Autodesk Fusion 360 part; units mm, degrees
sketch "Skizze1" plane through (0, 0, 0) normal (0, 1, 0) x (1, 0, 0)
  line L0 (0, 75) -> (0, -65)
  line L1 (0, -50) -> (0, 75)
  line L2 (-85, 0) -> (95, 0)
  line L3 (0, 0) -> (-37.5, 0)
  line L4 (-37.5, 0) -> (-37.5, -25)
  line L5 (-37.5, -25) -> (0, -25)
  line L6 (0, -25) -> (0, 0)
  line L7 (37.5, 0) -> (37.5, -25)
  line L8 (37.5, -25) -> (0, -25)
  line L9 (-37.5, 0) -> (-37.5, 25)
  line L10 (-37.5, 25) -> (0, 25)
  line L11 (37.5, 25) -> (0, 25)
  line L12 (37.5, 0) -> (37.5, 25)
  line L13 (-25.2075, -10.9903) -> (-29.8263, -11.0098)
  line L14 (-29.8263, -11.0098) -> (-32.1188, -15.0195)
  line L15 (-32.1188, -15.0195) -> (-29.7925, -19.0097)
  line L16 (-29.7925, -19.0097) -> (-25.1737, -18.9902)
  line L17 (-25.1737, -18.9902) -> (-22.8812, -14.9805)
  line L18 (-22.8812, -14.9805) -> (-25.2075, -10.9903)
  line L19 (22.8812, -14.9805) -> (25.2075, -10.9903)
  line L20 (25.2075, -10.9903) -> (29.8263, -11.0098)
  line L21 (29.8263, -11.0098) -> (32.1188, -15.0195)
  line L22 (32.1188, -15.0195) -> (29.7925, -19.0097)
  line L23 (29.7925, -19.0097) -> (25.1737, -18.9902)
  line L24 (25.1737, -18.9902) -> (22.8812, -14.9805)
  line L25 (-27.5, -15) -> (27.5, -15) construction
  line L26 (-37.5, -30) -> (-37.5, -55)
  line L27 (-37.5, -30) -> (-37.5, -5)
  line L28 (-37.5, -55) -> (0, -55)
  line L29 (37.5, -55) -> (0, -55)
  line L30 (37.5, -30) -> (37.5, -55)
  line L31 (37.5, -30) -> (37.5, -5)
  point P0 (-27.5, -15)
  point P1 (27.5, -15)
  point P2 (-27.5, -15)
  dimension "d1" = 37.5
  dimension "d2" = 25
  dimension "d7" = 10
  dimension "d8" = 55
  dimension "d9" = 4
extrude "Extrusion1" add sketch "Skizze1" along normal blind 10 contours L0 L1 L2 L11 L12 | L0 L1 L2 L3 L9 L10 | L0 L1 L2 L6 L7 L8 L31 | L0 L1 L2 L3 L4 L5 L6 L27 | L0 L1 L8 L29 L30 L31 | L0 L1 L5 L26 L27 L28 | L13 L14 L15 L16 L17 L18 | L19 L20 L21 L22 L23 L24
extrude "Extrusion2" cut sketch "Skizze1" along normal blind 4 contours L13 L14 L15 L16 L17 L18 | L19 L20 L21 L22 L23 L24
ref_plane "Arbeitsebene1" through (0, 10, 15) normal (0, 1, 0) x (0, 0, 1)
sketch "Skizze2" plane through (0, 10, 0) normal (0, 1, 0) x (1, 0, 0)
  line L0 (0, 75) -> (0, -65)
  line L1 (37.5, 25) -> (0, 25)
  line L2 (-27.5, -15) -> (27.5, -15)
  point P0 (-20, 15)
  point P1 (20, 15)
  point P2 (-20, -45)
  point P3 (20, -45)
  dimension "d15" = 40
  dimension "d16" = 10
hole "Bohrung1" at (-20, 10, -15) at (20, 10, -15) at (20, 10, 45) at (-20, 10, 45) direction (0, -1, 0) diameter 4.1 end through all countersink diameter 8 countersink angle 90
hole "Bohrung2" at (-27.5, 0, 15) direction (0, -1, 0) diameter 6 depth 12 tip angle 118
mirror "Spiegeln2" about plane through (0, 0, 0) normal (1, 0, 0) of "Bohrung2"
equation "d1 = ( 75 / 2 ) * 1 mm"
equation "d2 = ( 50 / 2 ) * 1 mm"
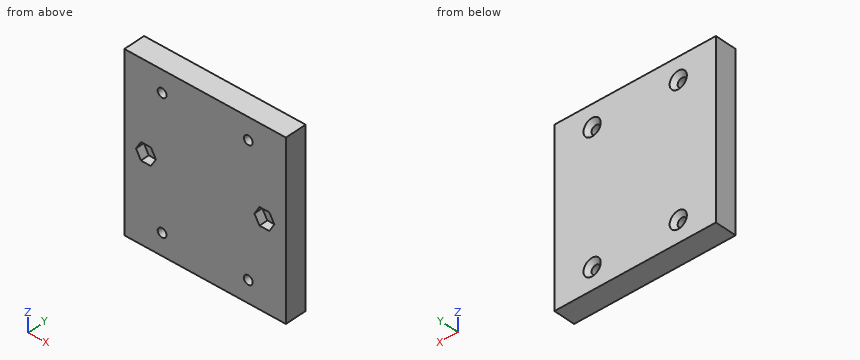
The model under review builds one solid part; all positions refer to its coordinate system, in mm. Coordinates: 2 decimals unless noted, no trailing zeros. Order: outer loops, then holes, each group sorted by start corner. A loop starts at its lowest first (then second) coordinate and runs counter-clockwise, first axis right, second up. Notation, with made-up numbers: (-27, 7) -> (-5, 7) arc R29 cw to (-5, 30) -> close; hole circle Ø2 at (11.5, 67). An arc over 180 degrees is marked (long way). Answer in a Markdown table with one row per item.
(1) Insertion check: pin 1 (6.5 mm diameter, centred on x = 20, z = 45, fed in from +Y); pin 2 (2.5 mm diameter, centred on x = -20, z = -15, fed in from +Y); pin 3 (4 mm diameter, centred on x = 27.5, z = 15, fed in from -Y); pin 4 (4.5 mm diameter, centred on x = 20, z = -15, fed in from +Y). Each pin has a flat end and moves straight along its axis. Give the tip position at first contact, or say it passes through.
Answers:
| item | result |
|---|---|
| pin 1 | y = 9.25 |
| pin 2 | through |
| pin 3 | y = 4 |
| pin 4 | y = 8.25 |
(2) Consider section B-B (y = 1.5). Write out the cut boundary in (x, z).
Answers:
| item | result |
|---|---|
| outline | (-37.5, -25) -> (37.5, -25) -> (37.5, 55) -> (-37.5, 55) -> close; hole (-32.12, 15.02) -> (-29.83, 11.01) -> (-25.21, 10.99) -> (-22.88, 14.98) -> (-25.17, 18.99) -> (-29.79, 19.01) -> close; hole circle Ø4.1 at (-20, -15); hole circle Ø4.1 at (-20, 45); hole circle Ø4.1 at (20, -15); hole circle Ø4.1 at (20, 45); hole (22.88, 14.98) -> (25.21, 10.99) -> (29.83, 11.01) -> (32.12, 15.02) -> (29.79, 19.01) -> (25.17, 18.99) -> close |
(3) Consider section A-A (x = 20). Write out the cut boundary in (y, z), plus the area to 3 significant figures.
Answers:
| item | result |
|---|---|
| outline | (0, -25) -> (10, -25) -> (10, -19) -> (8.05, -17.05) -> (0, -17.05) -> close; (0, -12.95) -> (8.05, -12.95) -> (10, -11) -> (10, 41) -> (8.05, 42.95) -> (0, 42.95) -> close; (0, 47.05) -> (8.05, 47.05) -> (10, 49) -> (10, 55) -> (0, 55) -> close |
| area | 710 mm² |
(4) Wall thickness on line 1 along Z through (x, y) = (-20, 2.5); line 2 along X through (y, z) = (2.25, 45); line 3 along X through (y, z) = (5, -13.5): over which ranges is each line inside the solid? List them lowest first.
Answers:
| item | result |
|---|---|
| line 1 | -25 to -17.05, -12.95 to 42.95, 47.05 to 55 |
| line 2 | -37.5 to -22.05, -17.95 to 17.95, 22.05 to 37.5 |
| line 3 | -37.5 to -21.4, -18.6 to 18.6, 21.4 to 37.5 |
(5) Consider section D-D (y = 9). Write out the cut boundary in (x, z).
Answers:
| item | result |
|---|---|
| outline | (-37.5, -25) -> (37.5, -25) -> (37.5, 55) -> (-37.5, 55) -> close; hole circle Ø6 at (-20, -15); hole circle Ø6 at (-20, 45); hole circle Ø6 at (20, -15); hole circle Ø6 at (20, 45) |
(6) Consider section C-C (z = -15). Write out the cut boundary in (x, y).
Answers:
| item | result |
|---|---|
| outline | (-37.5, 0) -> (-22.05, 0) -> (-22.05, 8.05) -> (-24, 10) -> (-37.5, 10) -> close; (-17.95, 0) -> (17.95, 0) -> (17.95, 8.05) -> (16, 10) -> (-16, 10) -> (-17.95, 8.05) -> close; (22.05, 0) -> (37.5, 0) -> (37.5, 10) -> (24, 10) -> (22.05, 8.05) -> close |
